Design review of the part shown in the three views and the two pictorial views. Dimensions are in mm from the part's minimum x, y and z. A direction names the side the tool comes from. Give positions to 0.01 mm unless a question says otherwise; leave off trailing zeros. Order: outer loops, then holes, each group sorted by start corner. A loop starts at its lowest first (then second) coordinate and runs counter-clockwise, first axis right, second up.
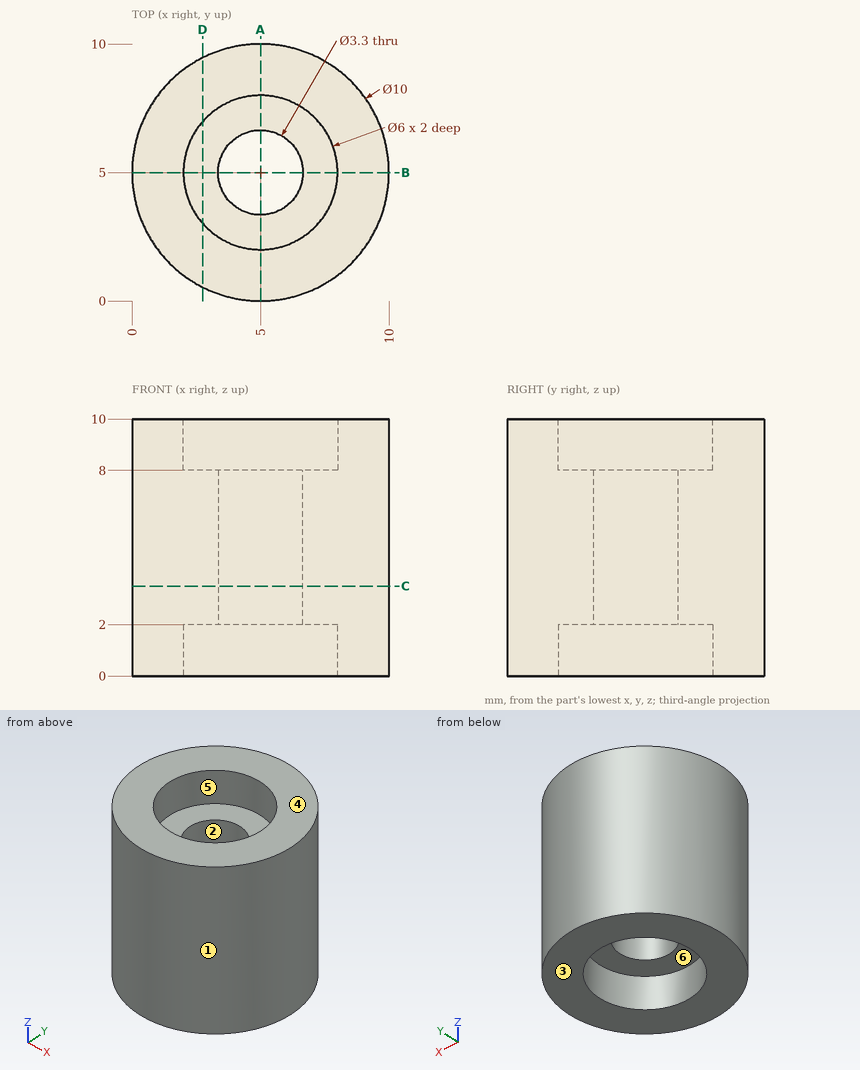
Item 1: Clearance check with flat-ended pins moving along their axes: pin 1 Ø3 at (y, z) = (4.5, 2) entering from -X; pin 2 Ø2 at (x, y) = (4, 4.5) entering from +Z; pin 3 Ø2 at (x, z) = (1, 4.5) entering from -Y; pin 4 Ø5 at (x, z) = (8, 5) entering from -Y. State where each tip first meets the part, or that it passes through.
Values found:
pin 1: stops at x = 0
pin 2: stops at z = 8
pin 3: stops at y = 1
pin 4: stops at y = 0.03
Item 2: Take a section at D-D (x = 2.75). Give the boundary of the cut face in (y, z).
Values found:
outline: (0.53, 0) - (3.02, 0) - (3.02, 2) - (6.98, 2) - (6.98, 0) - (9.47, 0) - (9.47, 10) - (6.98, 10) - (6.98, 8) - (3.02, 8) - (3.02, 10) - (0.53, 10) - close
Item 3: Draft analysis for pull direction Y (two halves, no side actions). For the marked faces 1, 2 and 3, state which applies: released by +Y, released by -Y, zero draft, split by the parting line, or undercut.
Values found:
face 1: split by the parting line
face 2: undercut
face 3: zero draft
Item 4: For line 1 (Y direction, x = 5, z = 5.9); line 2 (Y direction, x = 4, z = 8.75), list the stretches that pass through material, from the lowest coordinate up.
Values found:
line 1: y = 0 to 3.35, 6.65 to 10
line 2: y = 0.1 to 2.17, 7.83 to 9.9
Item 5: Take a section at A-A (x = 5). Give the boundary of the cut face in (y, z).
Values found:
outline: (0, 0) - (2, 0) - (2, 2) - (3.35, 2) - (3.35, 8) - (2, 8) - (2, 10) - (0, 10) - close; (6.65, 2) - (8, 2) - (8, 0) - (10, 0) - (10, 10) - (8, 10) - (8, 8) - (6.65, 8) - close
Item 6: Take a section at C-C (z = 3.5). Give the boundary of the cut face in (x, y).
Values found:
outline: circle Ø10 at (5, 5); hole circle Ø3.3 at (5, 5)
Item 7: For the marked faces 4, 5 and 6, list the 3-axis set-ups (+Z, -Z, +X, -X, +Y, -Y) from which the entire face can be reached by the end or side of a thin tool; tool diameter is ignored.
Values found:
face 4: +Z, +X, -X, +Y, -Y
face 5: +Z
face 6: -Z
